Part print with two shaded views. Sizes in mm from the minimum x, y, z corner. A direction names the side the tool comes from. Round coordinates to 2 decimals unless told otherwise and drop trailing zeros. Loops run counter-clockwise (first coordinate to the right, second up) from the corner with the lowest first, then second, coordinate; pieces in that order, holes last. Notation, with made-up numbers: (26.5, 61.25) - (34.5, 61.25) arc R30 ccw to (34.5, 83.25) - close; hole circle Ø1 at (68, 46.5). An arc over 180 degrees is marked (long way). Write each question's results on one line, items separated by ' | '. Start each with the question number.
(1) Cut at C-C, the plane x = 299.5. List the corners of the cut face in (y, z) (3 decimals).
(2) Cut at B-B, the plane y = 127. List the corners of the cut face in (x, z) (3 decimals), then the cut area to 3 significant figures.
(3) Cut at D-D, the plane y = 219.5. List the corners of the cut face in (x, z) (3 decimals).
(4) Mould opens along X. For the marked faces 1, 2, 3 and 4 say: released by +X, released by -X, zero draft, split by the parting line, or undercut.
(5) Drill centre lines: L1, parallel to X at y = 182.5, z = 27; L2, parallel to Y at x = 112, z = 25; L3, parallel to Y at x = 329.5, z = 42. Where is each one in solid material? Low to high.
(6) Tool access for the marked faces 5 and 6: list every direction of +Z, -Z, +X, -X, +Y, -Y with a clear straight run to the whole face (end or side of a thin tool).
(7) Cut at A-A, the plane z = 61. List the corners of the cut face in (x, y).
(8) Flat gauge pins, fed straight in: P1, Ø8, axis at x = 65.5, y = 194, coming from the +Z side; P2, Ø1.5, axis at y = 128, z = 15.5, coming from the -X side. Where does each tip first touch, or does it go through?
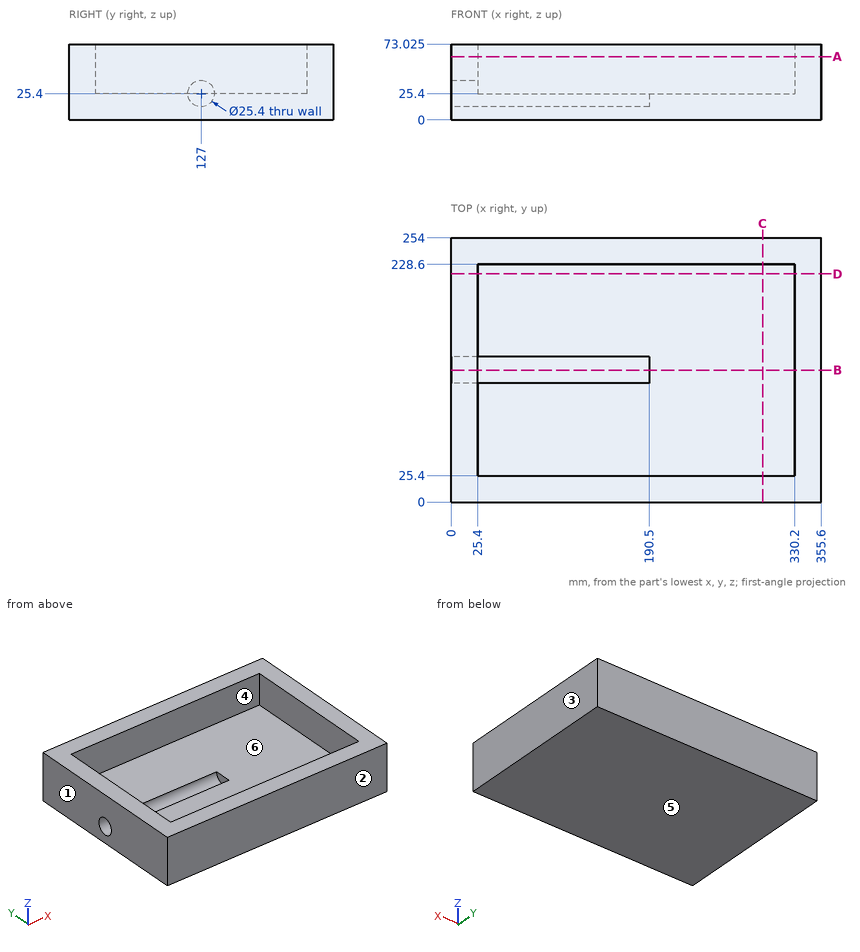
A:
1) outline: (0, 0) - (254, 0) - (254, 73.025) - (228.6, 73.025) - (228.6, 25.4) - (25.4, 25.4) - (25.4, 73.025) - (0, 73.025) - close
2) outline: (0, 0) - (355.6, 0) - (355.6, 73.025) - (330.2, 73.025) - (330.2, 25.4) - (190.5, 25.4) - (190.5, 12.7) - (0, 12.7) - close; (0, 38.1) - (25.4, 38.1) - (25.4, 73.025) - (0, 73.025) - close | area: 8,710 mm2
3) outline: (0, 0) - (355.6, 0) - (355.6, 73.025) - (330.2, 73.025) - (330.2, 25.4) - (25.4, 25.4) - (25.4, 73.025) - (0, 73.025) - close
4) face 1: released by -X | face 2: zero draft | face 3: released by +X | face 4: undercut
5) L1: 0 to 25.4, 330.2 to 355.6 | L2: 0 to 114.31, 139.69 to 254 | L3: 0 to 25.4, 228.6 to 254
6) face 5: -Z, +X, -X, +Y, -Y | face 6: +Z
7) outline: (0, 0) - (355.6, 0) - (355.6, 254) - (0, 254) - close; hole (25.4, 25.4) - (330.2, 25.4) - (330.2, 228.6) - (25.4, 228.6) - close
8) P1: z = 25.4 | P2: x = 190.5
